Read the model definition and answer for the solid it produces. Units are mm, in the model's axes. Face numbers are marked on the shaded views. A direction names the side the tool comes from. Give positions to 0.01 mm unless a question says otherwise; leave off trailing zeros. Write each loop counter-clockwise with the first axis right and the second up, starting at its lowest first coordinate (ties: lowest second). Pieces come first, ordered by that corner, then holes. Notation, with made-up numbers: M 83.25,-18.75 L 102.25,-18.75 A24 cw 102.25,-0.75 Z; hole C 34,-10 d2. An arc over 180 degrees is marked long. Put each result on its own line as item: value.
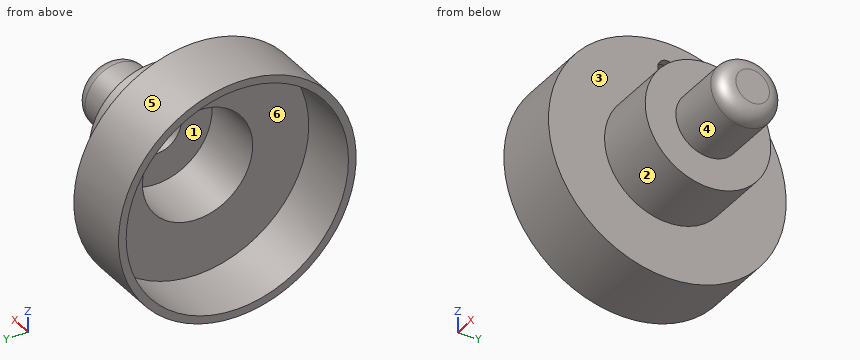
from build123d import *

# Parameters (mm, degrees)
F2_T = -2.54
F3_R = 5.08
F5_D = 6.35


with BuildPart() as f1:
    # F0 (on Front) → F1 (revolve)
    with BuildSketch(Plane.XZ):
        Polygon((0, 39.3052697182), (0, 0), (67.3264637589, 0), (67.3264637589, 10.6312446296), (44.1937856376, 10.6312446296), (44.1937856376, 20.7716822624), (23.1326818466, 20.7716822624), (23.1326818466, 39.3052697182), align=None)
    revolve(axis=Axis((33.6632318795, 0, 0), (1, 0, 0)))

    # F2
    f2_openings = [f1.faces().sort_by_distance(p)[0] for p in [
        (0, 0, 0),
    ]]
    offset(amount=F2_T, openings=f2_openings, kind=Kind.INTERSECTION)

    # F3
    f3_edges = [f1.edges().sort_by_distance(p)[0] for p in [
        (67.326464, 0, -10.631245),
    ]]
    fillet(f3_edges, radius=F3_R)

    # F5 (through all)
    with Locations(Plane.YZ.offset(23.1326818466)):
        with Locations((0, 30.2698779851)):
            Hole(F5_D / 2)


solid = f1.part
(1) For a pull along Y with two mould halves and no side action, classify the marked faces 1, 2 and 3 as +Y half, -Y half, draft (parallel to the pull), parting line (faces both ways), or undercut.
Result:
face 1: undercut
face 2: parting line
face 3: draft
(2) Section C-C on z = 0 is taken. Determine the outline of the cut face in (x, y), and give its area (3 significant figures).
Result:
outline: M 0,-39.31 L 23.13,-39.31 L 23.13,-20.77 L 44.19,-20.77 L 44.19,-10.63 L 62.25,-10.63 A5.08 ccw 67.33,-5.55 L 67.33,5.55 A5.08 ccw 62.25,10.63 L 44.19,10.63 L 44.19,20.77 L 23.13,20.77 L 23.13,39.31 L 0,39.31 L 0,36.77 L 20.59,36.77 L 20.59,18.23 L 41.65,18.23 L 41.65,8.09 L 64.79,8.09 L 64.79,-8.09 L 41.65,-8.09 L 41.65,-18.23 L 20.59,-18.23 L 20.59,-36.77 L 0,-36.77 Z
area: 518 mm²
(3) Which of the six approach directions +Z, -Z, +X, -X, +Y, -Y give full straight-line access (tool end or side, diameter ignored) to the marked faces 4, 5 and 6?
Result:
face 4: +X
face 5: +X, -X
face 6: -X
(4) Section B-B on x = 56.5 is taken. Determine the outline of the cut face in (y, z).
Result:
outline: C 0,0 d21.26; hole C 0,0 d16.18
(5) Given pin 1 Ø1 at (x, z) = (46, 14) entering from -Y; pin 2 Ø8 at (y, z) = (0, -0.5) entering from -X; pin 3 Ø10 at (x, z) = (20.5, -15.5) entering from +Y; pin 4 Ø12 at (x, y) = (9, -7.5) entering from +Z, each flat-ended and moving along its own axis, determine where each tip first touches the part or whether it passes through.
Result:
pin 1: passes through
pin 2: stops at x = 64.79
pin 3: stops at y = 37.88
pin 4: stops at z = 39.28
(6) Straight lines are drawn through the part: line 1 along Y through (x, z) = (51, 0); line 2 along Y through (x, z) = (4, 0); line 3 along X through (y, z) = (20.5, -23.5). For each, find the intervals that lie inside material, in ascending order. Write a range as from..to.
Result:
line 1: y = -10.63..-8.09, 8.09..10.63
line 2: y = -39.31..-36.77, 36.77..39.31
line 3: x = 20.59..23.13
(7) Section D-D on y = 13 is taken. Determine the outline of the cut face in (x, z), and give its area (3 significant figures).
Result:
outline: M 0,-37.09 L 23.13,-37.09 L 23.13,-16.2 L 44.19,-16.2 L 44.19,16.2 L 23.13,16.2 L 23.13,37.09 L 0,37.09 L 0,34.39 L 20.59,34.39 L 20.59,12.78 L 41.65,12.78 L 41.65,-12.78 L 20.59,-12.78 L 20.59,-34.39 L 0,-34.39 Z
area: 444 mm²
